Could you check a few things on this model? Use its own coordinates, in mm. Face numbers are marked on the shaded views. A direction names the side the tool comes from. Give positions to 0.01 mm unless a question says otherwise; leave off trailing zeros. Order: outer loops, then holes, each group sorted by start corner. A loop starts at its lowest first (then second) coordinate and runs counter-clockwise, first axis right, second up. Notation, with made-up numbers: (-2.5, -1) -> (52.5, -1) arc R22 cw to (52.5, 37) -> close; hole circle Ø6 at (75.5, 79). An arc over 180 degrees is marked (long way). One line per item, written item: value.
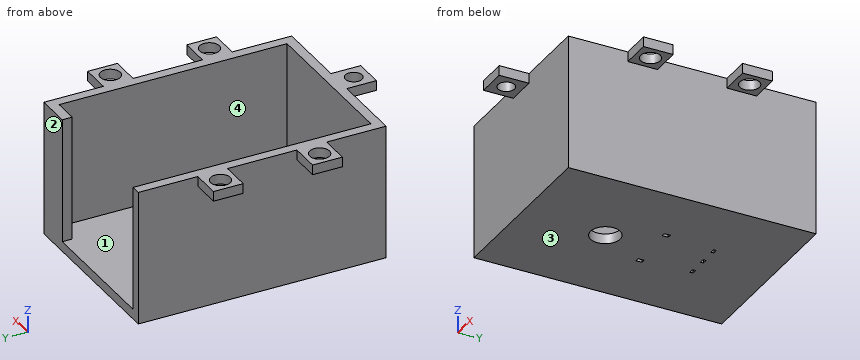
```python
from build123d import *

# Parameters (mm, degrees)
SKETCH1_W           = 36
SKETCH1_H           = 50
BOSS_EXTRUDE1_DEPTH = 27.2
CUT_EXTRUDE1_REACH  = 69.349
SKETCH2_R           = 3
SKETCH8_W           = 32
SKETCH8_H           = 46
CUT_EXTRUDE2_DEPTH  = 25.2
SKETCH12_W          = 1
SKETCH12_H          = 0.6
SKETCH12_W_2        = 0.8
SKETCH12_H_2        = 1.2
CUT_EXTRUDE3_DEPTH  = 25.2
SKETCH14_W          = 32
SKETCH14_H          = 25.2
CUT_EXTRUDE4_DEPTH  = 25.2
SKETCH16_W          = 5
SKETCH16_H          = 25.2
BOSS_EXTRUDE2_DEPTH = 2
SKETCH17_W          = 6
SKETCH17_H          = 6
BOSS_EXTRUDE3_DEPTH = 2
SKETCH18_R          = 2
CUT_EXTRUDE5_DEPTH  = 2
SKETCH20_W          = 6
SKETCH20_H          = 6
BOSS_EXTRUDE4_DEPTH = 2
SKETCH21_R          = 1.684389361
CUT_EXTRUDE6_DEPTH  = 2


with BuildPart() as part:
    # Sketch1 → Boss-Extrude1 (new body)
    with BuildSketch(Plane.XY):
        with Locations((18, 25)):
            Rectangle(SKETCH1_W, SKETCH1_H)
    extrude(amount=-BOSS_EXTRUDE1_DEPTH)

    # Sketch2 → Cut-Extrude1 (cut, up to next)
    with BuildSketch(Plane.XY, mode=Mode.PRIVATE) as cut_extrude1_sk1:
        with Locations((18, 33)):
            Circle(SKETCH2_R)
    cut_extrude1_tool1 = extrude(cut_extrude1_sk1.sketch, amount=-CUT_EXTRUDE1_REACH, mode=Mode.PRIVATE) & part.part
    add(cut_extrude1_tool1.solids().sort_by_distance((18, 33, 0))[0], mode=Mode.SUBTRACT)

    # Sketch8 → Cut-Extrude2 (cut)
    with BuildSketch(Plane.XY):
        with Locations((18, 25)):
            Rectangle(SKETCH8_W, SKETCH8_H)
    extrude(amount=-CUT_EXTRUDE2_DEPTH, mode=Mode.SUBTRACT)

    # Sketch12 → Cut-Extrude3 (cut)
    with BuildSketch(Plane(origin=(0, 0, -27.2), x_dir=(-1, 0, 0), z_dir=(0, 0, -1))):
        with Locations((-14, 13.25)):
            Rectangle(SKETCH12_W, SKETCH12_H)
        with Locations((-18, 13.25)):
            Rectangle(SKETCH12_W, SKETCH12_H)
        with Locations((-22, 13.25)):
            Rectangle(SKETCH12_W, SKETCH12_H)
        with Locations((-13, 23.35)):
            Rectangle(SKETCH12_W_2, SKETCH12_H_2)
        with Locations((-23, 23.35)):
            Rectangle(SKETCH12_W_2, SKETCH12_H_2)
    extrude(amount=-CUT_EXTRUDE3_DEPTH, mode=Mode.SUBTRACT)

    # Sketch14 → Cut-Extrude4 (cut)
    with BuildSketch(Plane.XZ):
        with Locations((18, -12.6)):
            Rectangle(SKETCH14_W, SKETCH14_H)
    extrude(amount=-CUT_EXTRUDE4_DEPTH, mode=Mode.SUBTRACT)

    # Sketch16 → Boss-Extrude2 (add)
    with BuildSketch(Plane(origin=(0, 0, 0), x_dir=(-1, 0, 0), z_dir=(0, -1, 0))):
        with Locations((-31.5, 12.6)):
            Rectangle(SKETCH16_W, SKETCH16_H)
    extrude(amount=-BOSS_EXTRUDE2_DEPTH)

    # Sketch20 → Boss-Extrude4 (add)
    with BuildSketch(Plane.XY):
        with Locations((18, 53)):
            Rectangle(SKETCH20_W, SKETCH20_H)
    extrude(amount=-BOSS_EXTRUDE4_DEPTH)

    # Sketch21 → Cut-Extrude6 (cut)
    with BuildSketch(Plane.XY):
        with Locations((18, 53)):
            Circle(SKETCH21_R)
    extrude(amount=-CUT_EXTRUDE6_DEPTH, mode=Mode.SUBTRACT)


with BuildPart() as body_2:
    # Sketch17 → Boss-Extrude3 (new body)
    with BuildSketch(Plane.XY):
        with Locations((39, 35)):
            Rectangle(SKETCH17_W, SKETCH17_H)
    extrude(amount=-BOSS_EXTRUDE3_DEPTH)

    # Sketch18 → Cut-Extrude5 (cut)
    with BuildSketch(Plane.XY):
        with Locations((39, 35)):
            Circle(SKETCH18_R)
    extrude(amount=-CUT_EXTRUDE5_DEPTH, mode=Mode.SUBTRACT)


with BuildPart() as body_3:
    # Mirror1: mirrored copy
    add(body_2.part.mirror(Plane(origin=(0, 25, 0), x_dir=(0, 0, 1), z_dir=(0, -1, 0))))


with BuildPart() as body_4:
    # Mirror2: mirrored copy
    add(body_2.part.mirror(Plane.ZY.offset(-18)))


with BuildPart() as body_5:
    # Mirror2 2: mirrored copy
    add(body_3.part.mirror(Plane.ZY.offset(-18)))


with BuildPart() as part_1:
    add(part.part)

    # Combine1: union body 3, body 2, body 4, body 5
    add(body_3.part)
    add(body_2.part)
    add(body_4.part)
    add(body_5.part)


with BuildPart() as body_2_2:
    # Mirror6: mirrored copy
    add(part_1.part.mirror(Plane(origin=(0, 0, 0), x_dir=(0, 0, 1), z_dir=(0, -1, 0))))


solid = body_2_2.part
```
1) For P1, Ø1.5, axis at x = 30, z = -9, coming from the -Y side; P2, Ø1.5, axis at x = 16, z = -5.5, coming from the +Y side; P3, Ø1.6, axis at y = -52, z = -1, coming from the -X side, each with a flat end and sliding along its axis, tell me the tip position at first contact or that it passes through.
Answer below:
P1: stops at y = -50
P2: stops at y = -48
P3: stops at x = 15
2) Suppose I cut it at A-A, the plane y = -53. Write out the boundary of the cut face in (x, z), then the cut area to 3 significant figures.
Answer below:
outline: (15, -2) -> (16.32, -2) -> (16.32, 0) -> (15, 0) -> close; (19.68, -2) -> (21, -2) -> (21, 0) -> (19.68, 0) -> close
area: 5.26 mm2
3) For the marked faces 3 and 4, which set-ups out of +Z, -Z, +X, -X, +Y, -Y let a thin tool reach every point of the face, with its end or its side?
Answer below:
face 3: -Z, +X, -X, +Y, -Y
face 4: +Z
4) Suppose I cut it at B-B, the plane x = 39. Write out the boundary of the cut face in (y, z), then the cut area to 3 significant figures.
Answer below:
outline: (-38, -2) -> (-37, -2) -> (-37, 0) -> (-38, 0) -> close; (-33, -2) -> (-32, -2) -> (-32, 0) -> (-33, 0) -> close; (-18, -2) -> (-17, -2) -> (-17, 0) -> (-18, 0) -> close; (-13, -2) -> (-12, -2) -> (-12, 0) -> (-13, 0) -> close
area: 8.00 mm2
5) If I drill on line 1 along X through (y, z) = (-35, -0.5); line 2 along Y through (x, z) = (18, -25.85); line 3 along Y through (x, z) = (32, -13.75), over which ranges is the centre line in solid material (lowest first)?
Answer below:
line 1: x = -6 to -5, -1 to 2, 34 to 37, 41 to 42
line 2: y = -50 to -36, -30 to -13.55, -12.95 to 0
line 3: y = -50 to -48, -2 to 0
6) Suppose I cut it at C-C, the plane y = -15. Write out the boundary of the cut face in (x, z).
Answer below:
outline: (-6, -2) -> (-5, -2) -> (-5, 0) -> (-6, 0) -> close; (-1, -2) -> (0, -2) -> (0, -27.2) -> (36, -27.2) -> (36, -2) -> (37, -2) -> (37, 0) -> (34, 0) -> (34, -25.2) -> (2, -25.2) -> (2, 0) -> (-1, 0) -> close; (41, -2) -> (42, -2) -> (42, 0) -> (41, 0) -> close
7) We'd pull the mould along X, two halves only. Please class the marked faces 1 and 2: +X half, -X half, draft (parallel to the pull), parting line (faces both ways), or undercut.
Answer below:
face 1: undercut
face 2: draft
8) Suppose I cut it at D-D, the plane z = -11.5. Write out the boundary of the cut face in (x, y), then the cut area to 3 significant figures.
Answer below:
outline: (0, -50) -> (36, -50) -> (36, 0) -> (29, 0) -> (29, -2) -> (34, -2) -> (34, -48) -> (2, -48) -> (2, 0) -> (0, 0) -> close
area: 274 mm2
